Check sheet for the drawn part. Datum: minimum x, y, z corner. Units: mm. Coordinates: 2 decimals unless noted, no trailing zeros. Write each loop counter-clockwise with the first axis right and the second up, starting at its lowest first coordinate (ties: lowest second). Pieces come first, ordered by that corner, then holes. Notation, with made-up numbers: (27, -28.75) -> (77, -28.75) arc R20 ccw to (77, -1.75) -> close; hole circle Ø8 at (5, 54). An arc over 180 degrees is marked (long way). Answer in a Markdown table with one row per item. Add a question column.
1. Mould release check, pull along Y, two halves, no side actions. Record for the marked faces 1, 2 and 3: pulls with the +Y half, pulls with the -Y half, needs draft (parallel to the pull), parting line crosses it, or undercut.
2. Cross-section at B-B on y = 7.5. Record the cut outline in (x, z) (1 decimal), and give its area (3 significant figures).
3. Scan lines: L1, parallel to Y at x = 1.7, z = 4.5 (1 decimal); L2, parallel to Z at x = 1.6, y = 1.5 (1 decimal); L3, parallel to Z at x = 0.95, y = 6.5. Record each from-to range of solid material in increasing order. Write a range as from..to.
4. Cross-section at D-D on y = 2. Record the cut outline in (x, z), and give its area (3 significant figures).
5. Cross-section at A-A on x = 1.15. Give the number of separate pieces and of enclosed holes in the cut face, and give its area (3 significant figures).
6. Cross-section at C-C on z = 4.5. Record the cut outline in (x, y) (1 decimal), and give its area (3 significant figures).
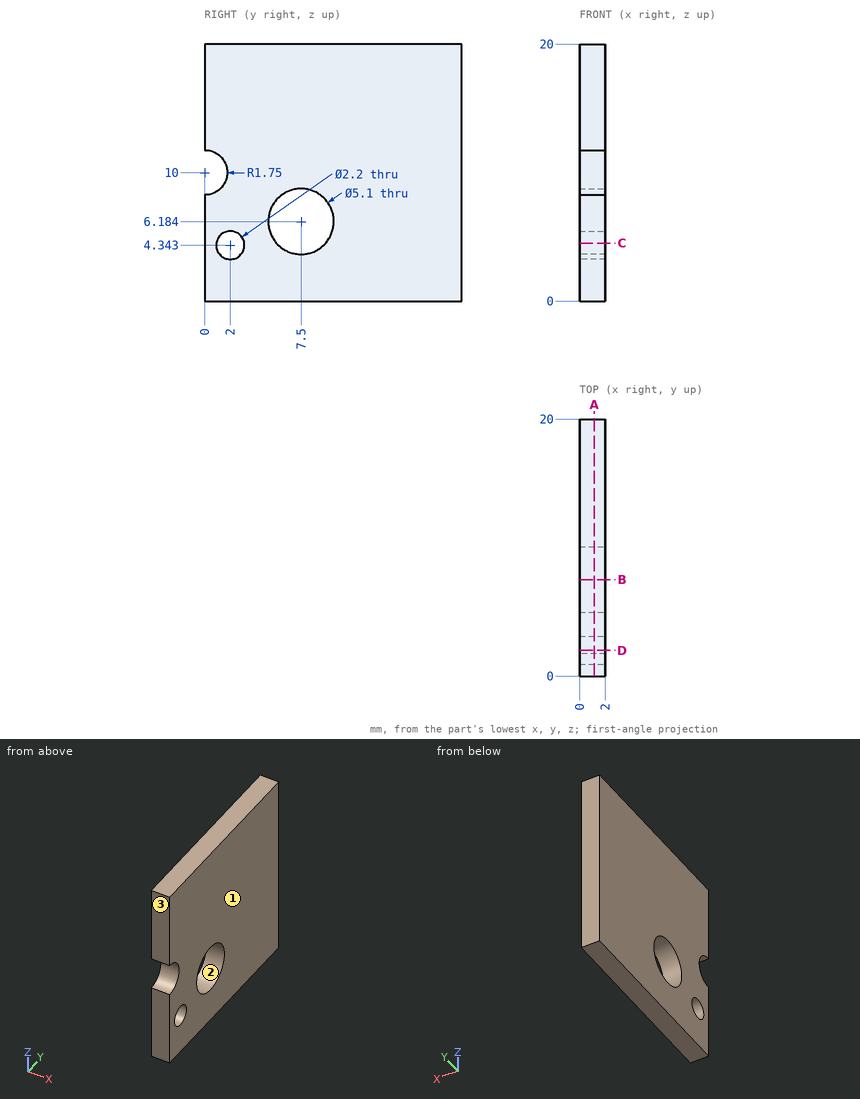
Results found:
| question | item | result |
|---|---|---|
| 1 | face 1 | needs draft |
| 1 | face 2 | undercut |
| 1 | face 3 | pulls with the -Y half |
| 2 | outline | (0, 0) -> (2, 0) -> (2, 3.6) -> (0, 3.6) -> close; (0, 8.7) -> (2, 8.7) -> (2, 20) -> (0, 20) -> close |
| 2 | area | 29.8 mm^2 |
| 3 | L1 | y = 0..0.9, 3.1..5.6, 9.4..20 |
| 3 | L2 | z = 0..3.4, 5.3..9.1, 10.9..20 |
| 3 | L3 | z = 0..3.84, 8.53..20 |
| 4 | outline | (0, 0) -> (2, 0) -> (2, 3.24) -> (0, 3.24) -> close; (0, 5.44) -> (2, 5.44) -> (2, 20) -> (0, 20) -> close |
| 4 | area | 35.6 mm^2 |
| 5 | separate pieces | 1 |
| 5 | enclosed holes | 2 |
| 5 | area | 371 mm^2 |
| 6 | outline | (0, 0) -> (2, 0) -> (2, 0.9) -> (0, 0.9) -> close; (0, 3.1) -> (2, 3.1) -> (2, 5.6) -> (0, 5.6) -> close; (0, 9.4) -> (2, 9.4) -> (2, 20) -> (0, 20) -> close |
| 6 | area | 28.0 mm^2 |
